CAD build for the part. Positions are in the model's coordinates, mm. Round coordinates to 2 decimals unless told otherwise and drop trailing zeros. Write each loop counter-clockwise with the first axis right and the second up, starting at its lowest first coordinate (ties: lowest second). Pieces come first, ordered by that corner, then holes. Notation, with made-up numbers: (63.5, 58) -> (120.5, 58) arc R24 ccw to (120.5, 78) -> close; hole circle Ø11 at (-34.5, 46.5). An arc over 180 degrees is marked (long way). Answer in a Markdown table with one row per item. Add a question column.
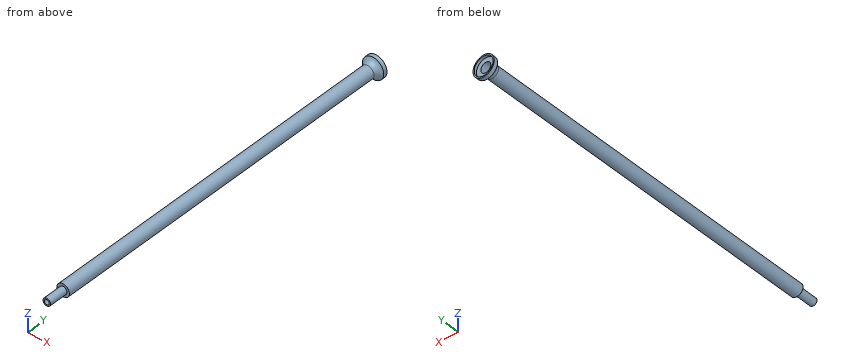
```python
from build123d import *

# Parameters (mm, degrees)
SHELL1_T           = -1
SKETCH2_R          = 2
CUT_EXTRUDE1_DEPTH = 300.241541234
FILLET1_R          = 5


with BuildPart() as part:
    # Sketch1 → Revolve1 (revolve)
    with BuildSketch(Plane(origin=(0, 0, 0), x_dir=(0, 0, -1), z_dir=(1, 0, 0)), mode=Mode.PRIVATE) as revolve1_sk:
        Polygon((0, 64.190330059), (8.5, 64.190330059), (8.5, 61.190330059), (5, 61.190330059), (5, -220.809669941), (3, -220.809669941), (3, -235.809669941), (0, -235.809669941), align=None)
    revolve(revolve1_sk.sketch.rotate(Axis((0, 68.843964237, 0), (0, -1, 0)), 180), axis=Axis((0, 68.843964237, 0), (0, -1, 0)))

    # Shell1
    shell1_openings = [part.faces().sort_by_distance(p)[0] for p in [
        (0, 64.190330059, 0),
    ]]
    offset(amount=SHELL1_T, openings=shell1_openings, kind=Kind.INTERSECTION)

    # Sketch2 → Cut-Extrude1 (cut, through all)
    with BuildSketch(Plane(origin=(0, -234.809669941, 0), x_dir=(1, 0, 0), z_dir=(0, 1, 0))):
        with Locations(Location((0, 0, 0), (0, 0, 270))):
            Circle(SKETCH2_R)
    extrude(amount=-CUT_EXTRUDE1_DEPTH, mode=Mode.SUBTRACT)

    # Fillet1
    # the kernel refuses this fillet: 5 mm, written as the material it adds along each edge
    with BuildSketch(Plane(origin=(0, 61.190330059, 0), x_dir=(0, 0, 1), z_dir=(1, 0, 0))) as fillet1_piece_1:
        with BuildLine():
            CenterArc((10, 4.769696007), FILLET1_R, 180, 72.542396876)
            Line((5, 4.769696007), (4.9, 4.769696007))
            Line((4.9, 4.769696007), (4.9, 0))
            Line((4.9, 0), (5, -0.1))
            ThreePointArc((5, -0.1), (6.75, -0.1), (8.47, -0.09539392))
            Line((8.47, -0.09539392), (8.5, 0))
        make_face()
    revolve(axis=Axis((0, 61.190330059, 0), (0, -1, 0)))


solid = part.part
```
Item 1: Saw through at A-A on y = 31. Give the cut face in (x, z), then the cut area to 3 significant figures.
Item 2: Pin check, flat tips, straight feed: pin 1 (9 mm diameter, centred on x = 0, z = 0, fed in from +Y); pin 2 (6 mm diameter, centred on y = -19, z = 0.5, fed in from -X); pin 3 (2 mm diameter, centred on x = 1.5, y = -182, fed in from +Z). Stop position of each tip, or through.
Item 3: Drill centre lines: probe 1 along X at (y, z) = (63.1, 0); probe 2 along X at (y, z) = (-43.5, 0); probe 3 along Y at (x, z) = (0.5, 2.5). Where is each one in solid material? Low to high.
Recorded:
| question | item | result |
|---|---|---|
| 1 | outline | circle Ø10 at (0, 0); hole circle Ø8 at (0, 0) |
| 1 | area | 28.3 mm2 |
| 2 | pin 1 | y = 62.19 |
| 2 | pin 2 | x = -5 |
| 2 | pin 3 | z = 4.97 |
| 3 | probe 1 | -8.5 to -7.5, 7.5 to 8.5 |
| 3 | probe 2 | -5 to -4, 4 to 5 |
| 3 | probe 3 | -235.81 to -219.81 |
